from build123d import *

# Parameters (mm, degrees)
SKETCH1_W           = 51.5
SKETCH1_H           = 20
BOSS_EXTRUDE1_DEPTH = 3.5
SKETCH2_W           = 12
SKETCH2_H           = 18
BOSS_EXTRUDE2_DEPTH = 3.5
FILLET1_R           = 1
FILLET2_R           = 1
SKETCH3_W           = 12
SKETCH3_H           = 18
BOSS_EXTRUDE3_DEPTH = 3.5
FILLET3_R           = 1
FILLET4_R           = 1
FILLET5_R           = 1
FILLET6_R           = 1
FILLET7_R           = 1
FILLET8_R           = 1
FILLET9_R           = 1
FILLET10_R          = 1
FILLET11_R          = 1
FILLET12_R          = 1
SKETCH4_W           = 12
SKETCH4_H           = 1.95
BOSS_EXTRUDE4_DEPTH = 7
SKETCH5_W           = 12
SKETCH5_H           = 1.95
BOSS_EXTRUDE5_DEPTH = 7
FILLET13_R          = 1
FILLET14_R          = 1
FILLET15_R          = 1
FILLET16_R          = 1
FILLET17_R          = 1
SKETCH8_W           = 16.25
SKETCH8_H           = 25.726511914
BOSS_EXTRUDE6_DEPTH = 11.42
FILLET21_R          = 2
FILLET22_R          = 2
FILLET23_R          = 2


with BuildPart() as part:
    # Sketch1 → Boss-Extrude1 (new body)
    with BuildSketch(Plane.XY):
        Rectangle(SKETCH1_W, SKETCH1_H)
    extrude(amount=BOSS_EXTRUDE1_DEPTH)

    # Sketch2 → Boss-Extrude2 (add)
    with BuildSketch(Plane(origin=(0, 10, 0), x_dir=(1, 0, 0), z_dir=(0, 1, 0))):
        with Locations((11.75, -10.75)):
            Rectangle(SKETCH2_W, SKETCH2_H)
    extrude(amount=BOSS_EXTRUDE2_DEPTH)

    # Fillet1
    fillet1_edges = [part.edges().sort_by_distance(p)[0] for p in [
        (11.75, 10, 1.75),
    ]]
    fillet(fillet1_edges, radius=FILLET1_R)

    # Fillet2
    fillet2_edges = [part.edges().sort_by_distance(p)[0] for p in [
        (11.75, 10, 3.5),
    ]]
    fillet(fillet2_edges, radius=FILLET2_R)

    # Sketch3 → Boss-Extrude3 (add)
    with BuildSketch(Plane(origin=(0, -10, 0), x_dir=(-1, 0, 0), z_dir=(0, -1, 0))):
        with Locations((-11.75, -10.75)):
            Rectangle(SKETCH3_W, SKETCH3_H)
    extrude(amount=BOSS_EXTRUDE3_DEPTH)

    # Fillet3
    fillet3_edges = [part.edges().sort_by_distance(p)[0] for p in [
        (11.75, -10, 1.75),
    ]]
    fillet(fillet3_edges, radius=FILLET3_R)

    # Fillet4
    fillet4_edges = [part.edges().sort_by_distance(p)[0] for p in [
        (11.75, -10, 3.5),
    ]]
    fillet(fillet4_edges, radius=FILLET4_R)

    # Fillet5
    fillet5_edges = [part.edges().sort_by_distance(p)[0] for p in [
        (17.75, 10, 2.125),
    ]]
    fillet(fillet5_edges, radius=FILLET5_R)

    # Fillet6
    fillet6_edges = [part.edges().sort_by_distance(p)[0] for p in [
        (5.75, 10, 2.125),
    ]]
    fillet(fillet6_edges, radius=FILLET6_R)

    # Fillet7
    fillet7_edges = [part.edges().sort_by_distance(p)[0] for p in [
        (17.75, 10, 3.5),
    ]]
    fillet(fillet7_edges, radius=FILLET7_R)

    # Fillet8
    fillet8_edges = [part.edges().sort_by_distance(p)[0] for p in [
        (5.75, 10, 3.5),
    ]]
    fillet(fillet8_edges, radius=FILLET8_R)

    # Fillet9
    fillet9_edges = [part.edges().sort_by_distance(p)[0] for p in [
        (5.75, -10, 2.125),
    ]]
    fillet(fillet9_edges, radius=FILLET9_R)

    # Fillet10
    fillet10_edges = [part.edges().sort_by_distance(p)[0] for p in [
        (5.75, -10, 3.5),
    ]]
    fillet(fillet10_edges, radius=FILLET10_R)

    # Fillet11
    fillet11_edges = [part.edges().sort_by_distance(p)[0] for p in [
        (17.75, -10, 2.125),
    ]]
    fillet(fillet11_edges, radius=FILLET11_R)

    # Fillet12
    fillet12_edges = [part.edges().sort_by_distance(p)[0] for p in [
        (17.75, -10, 3.5),
    ]]
    fillet(fillet12_edges, radius=FILLET12_R)

    # Sketch4 → Boss-Extrude4 (add)
    with BuildSketch(Plane(origin=(0, -10, 0), x_dir=(1, 0, 0), z_dir=(0, 1, 0))):
        with Locations((11.75, -18.775)):
            Rectangle(SKETCH4_W, SKETCH4_H)
    extrude(amount=BOSS_EXTRUDE4_DEPTH)

    # Sketch5 → Boss-Extrude5 (add)
    with BuildSketch(Plane(origin=(0, 10, 0), x_dir=(-1, 0, 0), z_dir=(0, -1, 0))):
        with Locations((-11.75, -18.775)):
            Rectangle(SKETCH5_W, SKETCH5_H)
    extrude(amount=BOSS_EXTRUDE5_DEPTH)

    # Fillet13
    fillet13_edges = [part.edges().sort_by_distance(p)[0] for p in [
        (11.75, 10, 17.8),
    ]]
    fillet(fillet13_edges, radius=FILLET13_R)

    # Fillet14
    fillet14_edges = [part.edges().sort_by_distance(p)[0] for p in [
        (11.75, 13.5, 19.75),
    ]]
    fillet(fillet14_edges, radius=FILLET14_R)

    # Fillet15
    fillet15_edges = [part.edges().sort_by_distance(p)[0] for p in [
        (11.75, 13.5, 1.75),
    ]]
    fillet(fillet15_edges, radius=FILLET15_R)

    # Fillet16
    fillet16_edges = [part.edges().sort_by_distance(p)[0] for p in [
        (11.75, -13.5, 19.75),
    ]]
    fillet(fillet16_edges, radius=FILLET16_R)

    # Fillet17
    fillet17_edges = [part.edges().sort_by_distance(p)[0] for p in [
        (11.75, -10, 17.8),
    ]]
    fillet(fillet17_edges, radius=FILLET17_R)

    # Sketch8 → Boss-Extrude6 (add)
    with BuildSketch(Plane(origin=(0, 0, 0), x_dir=(-1, 0, 0), z_dir=(0, 0, -1))):
        with Locations((17.625, -2.863255957)):
            Rectangle(SKETCH8_W, SKETCH8_H)
    extrude(amount=BOSS_EXTRUDE6_DEPTH)

    # Fillet21
    fillet21_edges = [part.edges().sort_by_distance(p)[0] for p in [
        (-9.5, 0, 0),
    ]]
    fillet(fillet21_edges, radius=FILLET21_R)

    # Fillet22
    fillet22_edges = [part.edges().sort_by_distance(p)[0] for p in [
        (-17.625, -10, 0),
    ]]
    fillet(fillet22_edges, radius=FILLET22_R)

    # Fillet23
    fillet23_edges = [part.edges().sort_by_distance(p)[0] for p in [
        (-9.5, -10, 0),
    ]]
    fillet(fillet23_edges, radius=FILLET23_R - 0.0001)  # a hair under: the kernel refuses the full size


solid = part.part
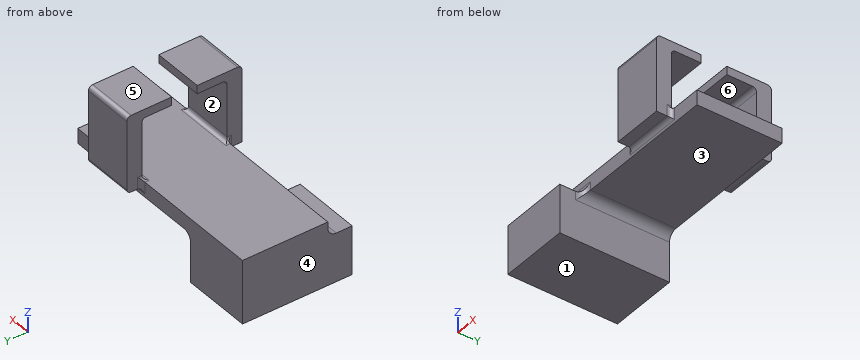
CAD build for the part. Positions are in the model's coordinates, mm. Face numbers are marked on the shaded views. A direction names the side the tool comes from. Give positions to 0.01 mm unless a question says otherwise; leave off trailing zeros. Write each loop counter-clockwise with the first axis right and the second up, starting at its lowest first coordinate (ties: lowest second). Pieces come first, ordered by that corner, then holes. Notation, with made-up numbers: (56, 67) -> (62, 67) arc R10 cw to (62, 75) -> close; hole circle Ø3 at (-35.75, 52). An arc over 180 degrees is marked (long way). Return JSON: item names as keys, results as strings.
Item 1: Drill centre lines: probe 1 along Z at (x, y) = (16, -3.5); probe 2 along Y at (x, z) = (15, 16.5); probe 3 along Z at (x, y) = (14.5, -2.25). Where is each one in solid material? Low to high.
Answer below:
{"probe 1": "z = 0 to 3.5, 17.8 to 19.75", "probe 2": "y = -13.5 to -10, 10 to 13.5", "probe 3": "z = 0 to 3.5"}
Item 2: Band-saw the part on D-D (y = 6). List the corners of the cut face in (x, z), then the cut area to 3 significant figures.
Answer below:
{"outline": "(-25.75, -11.42) -> (-9.5, -11.42) -> (-9.5, -2) arc R2 cw to (-7.5, 0) -> (25.75, 0) -> (25.75, 3.5) -> (-25.75, 3.5) -> close; (5.75, 17.8) -> (17.75, 17.8) -> (17.75, 19.75) -> (5.75, 19.75) -> close", "area": "390 mm2"}
Item 3: Band-saw the part on B-B (x = -16). List the corners of the cut face in (y, z), then the cut area to 3 significant figures.
Answer below:
{"outline": "(-15.73, -11.42) -> (10, -11.42) -> (10, 3.5) -> (-10, 3.5) -> (-10, 2) arc R2 cw to (-12, 0) -> (-15.73, 0) -> close", "area": "365 mm2"}
Item 4: Drop flat-ended pins along their axis: pin 1 (8.5 mm diameter, centred on y = -6.5, z = 11.5, fed in from -X); pin 2 (5 mm diameter, centred on y = 8, z = 10.5, fed in from +X); pin 3 (10 mm diameter, centred on x = 1.5, y = 10.5, fed in from -Z); pin 4 (3 mm diameter, centred on y = -11, z = 2, fed in from -X). Give the stop position or say it passes through.
Answer below:
{"pin 1": "stops at x = 5.75", "pin 2": "stops at x = 17.75", "pin 3": "stops at z = 0", "pin 4": "stops at x = -25.75"}
Item 5: Tool access for the marked faces 1, 2 and 3: list every direction of +Z, -Z, +X, -X, +Y, -Y with a clear straight run to the whole face (end or side of a thin tool).
Answer below:
{"face 1": "-Z, +X, -X, +Y, -Y", "face 2": "+X, -X", "face 3": "-Z, +X, +Y, -Y"}
Item 6: Band-saw the part on A-A (z = 8.5). List the corners of the cut face in (x, y), then the cut area to 3 significant figures.
Answer below:
{"outline": "(5.75, -13.5) -> (17.75, -13.5) -> (17.75, -10) -> (5.75, -10) -> close; (5.75, 10) -> (17.75, 10) -> (17.75, 13.5) -> (5.75, 13.5) -> close", "area": "84.0 mm2"}
Item 7: Band-saw the part on C-C (y = 2.25). List the corners of the cut face in (x, z), then the cut area to 3 significant figures.
Answer below:
{"outline": "(-25.75, -11.42) -> (-9.5, -11.42) -> (-9.5, -2) arc R2 cw to (-7.5, 0) -> (25.75, 0) -> (25.75, 3.5) -> (-25.75, 3.5) -> close", "area": "367 mm2"}
Item 8: Two-plate mould, pull along Z, no slides. Class the marked faces 4, 5 and 6: +Z half, -Z half, draft (parallel to the pull), parting line (faces both ways), or undercut.
Answer below:
{"face 4": "draft", "face 5": "+Z half", "face 6": "undercut"}
